Check sheet for the drawn part. Datum: minimum x, y, z corner. Units: mm. A direction names the side the tool comes from. Round coordinates to 2 decimals unless told otherwise and drop trailing zeros. Order: outer loops, then holes, each group sorted by start corner. A loop starts at its lowest first (then second) coordinate and runs counter-clockwise, first axis right, second up. Notation, with made-up numbers: M -39.5,-17.5 L 17.5,-17.5 A16 cw 17.5,8.5 Z; hole C 24.25,49.25 d2. An arc over 180 degrees is marked long. Answer as a JSON object with one key per item and string values. Group by question number.
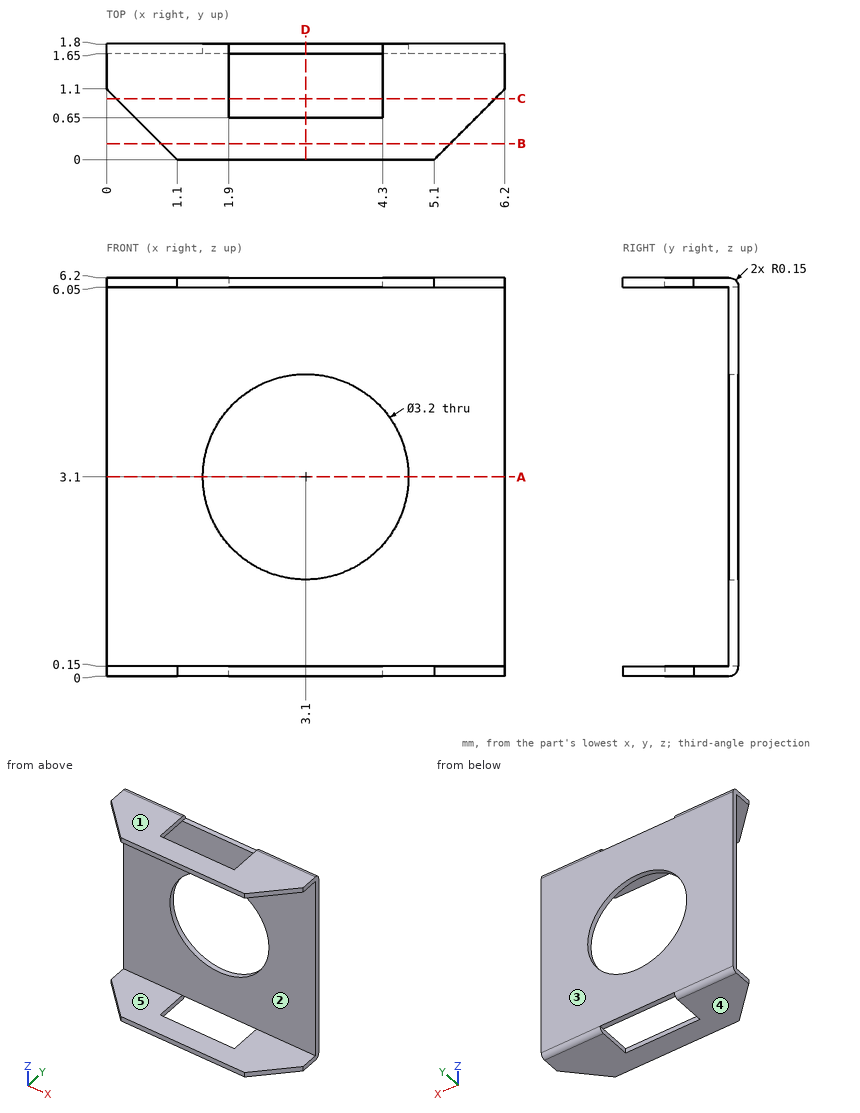
1) Sectioned sample at C-C (y = 0.95). Record the boundary of the cut face in (x, z).
2) Sectioned sample at B-B (y = 0.25). Record the boundary of the cut face in (x, z).
3) Set-up check for the marked faces 1 and 2: record each of +Z, -Z, +X, -X, +Y, -Y from which the full face is reachable in a straight line by a thin tool's end or side.
4) Thickness scan on line 1 along Z through (x, y) = (3.1, 1.75). Record the ranges inside material, lowest first. Write a range as [from, to].
5) Sectioned sample at D-D (x = 3.1). Record the boundary of the cut face in (y, z).
6) Release check for a two-part mould opening along Z. For the marked faces 3, 4 and 5 record: +Z half, -Z half, draft (parallel to the pull), parting line (faces both ways), or undercut.
7) Sectioned sample at A-A (z = 3.1). Record the boundary of the cut face in (x, y).
8) Go/stop test with a flat-tipped pin: P1, Ø1, axis at x = 3.5, z = 5, coming from the -Y side. Record where the tip stops, or that it passes through.
Final values:
{
 "1": {"outline": "M 0.15,0 L 1.9,0 L 1.9,0.15 L 0.15,0.15 Z; M 0.15,6.05 L 1.9,6.05 L 1.9,6.2 L 0.15,6.2 Z; M 4.3,0 L 6.05,0 L 6.05,0.15 L 4.3,0.15 Z; M 4.3,6.05 L 6.05,6.05 L 6.05,6.2 L 4.3,6.2 Z"},
 "2": {"outline": "M 0.85,0 L 5.35,0 L 5.35,0.15 L 0.85,0.15 Z; M 0.85,6.05 L 5.35,6.05 L 5.35,6.2 L 0.85,6.2 Z"},
 "3": {"face 1": "+Z, +X, -X, +Y, -Y", "face 2": "+X, -X, -Y"},
 "4": {"line 1": "z = [0.15, 1.5], [4.7, 6.05]"},
 "5": {"outline": "M 0,0 L 0.65,0 L 0.65,0.15 L 0,0.15 Z; M 0,6.05 L 0.65,6.05 L 0.65,6.2 L 0,6.2 Z; M 1.65,0.15 L 1.8,0.15 L 1.8,1.5 L 1.65,1.5 Z; M 1.65,4.7 L 1.8,4.7 L 1.8,6.05 L 1.65,6.05 Z"},
 "6": {"face 3": "draft", "face 4": "-Z half", "face 5": "undercut"},
 "7": {"outline": "M 0,1.65 L 1.5,1.65 L 1.5,1.8 L 0,1.8 Z; M 4.7,1.65 L 6.2,1.65 L 6.2,1.8 L 4.7,1.8 Z"},
 "8": {"P1": "stops at y = 1.65"}
}
